from build123d import *

# Parameters (mm, degrees)
ESQUISSE1_R             = 11.5
ESQUISSE1_R_2           = 1.75
BOSS_EXTRU_1_DEPTH      = 7
ESQUISSE2_W             = 20
ESQUISSE2_H             = 3
ESQUISSE2_W_2           = 3
ESQUISSE2_H_2           = 20
BOSS_EXTRU_2_DEPTH      = 15
ESQUISSE3_W             = 20
ESQUISSE3_H             = 17
BOSS_EXTRU_3_DEPTH      = 30
ESQUISSE4_R             = 2.5
ENL_V_MAT_EXTRU_1_DEPTH = 60.651592602
ESQUISSE5_R             = 4.5
ENL_V_MAT_EXTRU_2_DEPTH = 5
ENL_V_MAT_EXTRU_3_DEPTH = 10
CONG_1_R                = 3
CONG_2_R                = 3
CHANFREIN1_SIZE         = 1


with BuildPart() as part:
    # Esquisse1 → Boss.-Extru.1 (new body)
    with BuildSketch(Plane.XY):
        Polygon((-17.749999999, 21.249999999), (-21.249999999, 17.749999999), (-21.249999999, -17.749999999), (-17.749999999, -21.250000001), (17.749999999, -21.250000001), (21.249999999, -17.749999999), (21.249999999, 17.749999999), (17.749999999, 21.249999999), align=None)
        Circle(ESQUISSE1_R, mode=Mode.SUBTRACT)
        with Locations((-15.5, 15.5)):
            Circle(ESQUISSE1_R_2, mode=Mode.SUBTRACT)
        with Locations((15.5, 15.5)):
            Circle(ESQUISSE1_R_2, mode=Mode.SUBTRACT)
        with Locations((15.5, -15.5)):
            Circle(ESQUISSE1_R_2, mode=Mode.SUBTRACT)
        with Locations((-15.5, -15.5)):
            Circle(ESQUISSE1_R_2, mode=Mode.SUBTRACT)
    extrude(amount=BOSS_EXTRU_1_DEPTH)

    # Esquisse2 → Boss.-Extru.2 (add)
    with BuildSketch(Plane(origin=(0, 0, 0), x_dir=(-1, 0, 0), z_dir=(0, 0, -1))):
        with Locations((0, 22.749999999)):
            Rectangle(ESQUISSE2_W, ESQUISSE2_H)
        with Locations((22.749999999, 0)):
            Rectangle(ESQUISSE2_W_2, ESQUISSE2_H_2)
        with Locations((-22.749999999, 0)):
            Rectangle(ESQUISSE2_W_2, ESQUISSE2_H_2)
    extrude(amount=-BOSS_EXTRU_2_DEPTH)

    # Esquisse3 → Boss.-Extru.3 (add)
    with BuildSketch(Plane(origin=(0, 0, 0), x_dir=(-1, 0, 0), z_dir=(0, 0, -1))):
        with Locations((0, -29.750000001)):
            Rectangle(ESQUISSE3_W, ESQUISSE3_H)
    extrude(amount=-BOSS_EXTRU_3_DEPTH)

    # Esquisse4 → Enlèv. mat.-Extru.1 (cut, through all)
    with BuildSketch(Plane(origin=(0, -21.250000001, 0), x_dir=(1, 0, 0), z_dir=(0, 1, 0))):
        with Locations(Location((0, -22, 0), (0, 0, 270))):
            Circle(ESQUISSE4_R)
    extrude(amount=-ENL_V_MAT_EXTRU_1_DEPTH, mode=Mode.SUBTRACT)

    # Esquisse5 → Enlèv. mat.-Extru.2 (cut)
    with BuildSketch(Plane(origin=(0, -21.250000001, 0), x_dir=(1, 0, 0), z_dir=(0, 1, 0))):
        with Locations(Location((0, -22, 0), (0, 0, 270))):
            Circle(ESQUISSE5_R)
    extrude(amount=-ENL_V_MAT_EXTRU_2_DEPTH, mode=Mode.SUBTRACT)

    # Esquisse6 → Enlèv. mat.-Extru.3 (cut)
    with BuildSketch(Plane(origin=(0, -38.250000001, 0), x_dir=(-1, 0, 0), z_dir=(0, -1, 0))):
        with BuildLine():
            Line((3.010398645, -19), (-3.010398645, -19))
            ThreePointArc((-3.010398645, -19), (0, -26.25), (3.010398645, -19))
        make_face()
    extrude(amount=-ENL_V_MAT_EXTRU_3_DEPTH, mode=Mode.SUBTRACT)

    # Congé1
    cong_1_edges = [part.edges().sort_by_distance(p)[0] for p in [
        (-21.249999999, -10, 3.5),
        (-21.249999999, 10, 3.5),
        (-10, 21.249999999, 3.5),
        (10, 21.249999999, 3.5),
        (21.249999999, 10, 3.5),
        (21.249999999, -10, 3.5),
        (-10, -38.250000001, 15),
        (10, -38.250000001, 15),
        (10, -21.250000001, 3.5),
        (-10, -21.250000001, 3.5),
    ]]
    fillet(cong_1_edges, radius=CONG_1_R - 0.0001)  # a hair under: the kernel refuses the full size

    # Congé2
    cong_2_edges = [part.edges().sort_by_distance(p)[0] for p in [
        (-10, -28.250050001, 30),
        (0, -38.250000001, 30),
        (9.121349633, -37.371349634, 30),
        (-9.121349633, -37.371349634, 30),
        (10, -28.250050001, 30),
    ]]
    fillet(cong_2_edges, radius=CONG_2_R - 0.0001)  # a hair under: the kernel refuses the full size

    # Chanfrein1
    chanfrein1_edges = [part.edges().sort_by_distance(p)[0] for p in [
        (-11.5, 0, 7),
        (0, 21.249999999, 15),
        (-21.249999999, 0, 15),
        (21.249999999, 0, 15),
    ]]
    chamfer(chanfrein1_edges, length=CHANFREIN1_SIZE)


solid = part.part
Input: part model. Units: mm. Frame: model coordinates. A direction names the side the tool comes from. Give positions to 0.01 mm unless a question says otherwise; leave off trailing zeros. Write each loop counter-clockwise with the first axis right and the second up, starting at its lowest first coordinate (ties: lowest second). Pieces come first, ordered by that corner, then holes.
Q1. Section C-C, the plane y = 0. Output: boundary loops of the cut face in (x, z).
Q2. First-contact query: P1, Ø11, axis at y = -30.5, z = 11.5, coming from the -X side; P2, Ø5, axis at y = 15, z = 3.5, coming from the +X side; P3, Ø7, axis at x = -2, z = 23.5, coming from the +Y side. Flat tips, straight axial feed; report the tip coordinate or a pass-through.
Q3. Material intervals for probe 1 along Y at (x, z) = (15.5, 2.5); probe 2 along X at (y, z) = (-34.25, 22); probe 3 along X at (y, z) = (-27.75, 22), sorted ascending.
Q4. Pull-direction query (Y, two-part tool) for faces 4 (the face through (-0.1, -37.35, 29.14)), 5 (the face through (0, 21.25, 10)), 6 (the face through (-23, 0, 15)), 7 (the face through (20, 19, 3)); classes: pulls with the +Y half, pulls with the -Y half, needs draft (parallel to the pull), parting line crosses it, or undercut.
Q5. Section A-A, the plane y = 15.5. Output: boundary loops of the cut face in (x, z).
Q6. Section B-B, the plane z = 22. Output: boundary loops of the cut face in (x, y), plus the area to 3 significant figures.
Q7. Set-up query: faces 1 (the face through (-15, -21.25, 3)), 2 (the face through (15, -21.25, 3)), 3 (the face through (-23, -10, 11)). Return all of +Z, -Z, +X, -X, +Y, -Y with unobstructed straight access to the full face (end or side cutting, diameter ignored); none if empty.
Filled in:
1. outline: (-24.25, 0) - (-11.5, 0) - (-11.5, 6) - (-12.5, 7) - (-21.25, 7) - (-21.25, 14) - (-22.25, 15) - (-24.25, 15) - close; (11.5, 0) - (24.25, 0) - (24.25, 15) - (22.25, 15) - (21.25, 14) - (21.25, 7) - (12.5, 7) - (11.5, 6) - close
2. P1: stops at x = -10
2. P2: stops at x = 21.29
2. P3: stops at y = -21.25
3. probe 1: y = -21.25 to -17.25, -13.75 to 13.75, 17.25 to 21.25
3. probe 2: x = -10 to -4.25, 4.25 to 10
3. probe 3: x = -10 to -2.5, 2.5 to 10
4. face 4: pulls with the -Y half
4. face 5: undercut
4. face 6: needs draft
4. face 7: pulls with the +Y half
5. outline: (-21.25, 0) - (-17.25, 0) - (-17.25, 7) - (-21.25, 7) - close; (-13.75, 0) - (13.75, 0) - (13.75, 7) - (-13.75, 7) - close; (17.25, 0) - (21.25, 0) - (21.25, 7) - (17.25, 7) - close
6. outline: (-10, -35.25) arc R3 ccw to (-7, -38.25) - (-4.25, -38.25) - (-4.25, -28.25) - (-2.5, -28.25) - (-2.5, -26.25) - (-4.5, -26.25) - (-4.5, -21.25) - (-10, -21.25) - close; (2.5, -28.25) - (4.25, -28.25) - (4.25, -38.25) - (7, -38.25) arc R3 ccw to (10, -35.25) - (10, -21.25) - (4.5, -21.25) - (4.5, -26.25) - (2.5, -26.25) - close
6. area: 196 mm2
7. face 1: +Z, -Z, -X, -Y
7. face 2: +Z, -Z, +X, -Y
7. face 3: +Z, +X, -X, -Y
